Geometry: final body of the model. Coordinates: model frame, mm. Face numbers are marked on the shaded views. Give positions to 0.01 mm unless a question says otherwise; leave off trailing zeros. Order: outer loops, then holes, each group sorted by start corner. A loop starts at its lowest first (then second) coordinate and runs counter-clockwise, first axis right, second up. Notation, with made-up numbers: (39, -2.75) - (47, -2.75) arc R12 ccw to (47, 6.25) - close; hole circle Ø6 at (-28.75, 81.25). An arc over 180 degrees is marked (long way). Put each result on its own line as item: value. Start each with the question number.
1. Section A-A on x = 0. Return the cut outline in (y, z).
2. Section B-B on z = 0. Return the cut outline in (x, y).
3. Mould query, pull axis Z, two halves, no side actions, for the marked faces 1, 2 and 3. Classes: pulls with the +Z half, pulls with the -Z half, needs draft (parallel to the pull), parting line crosses it, or undercut.
4. Ray query, line 1 along X through (y, z) = (9.75, 0); line 2 along Y through (x, z) = (-4.5, 17); line 3 along Z through (x, y) = (30, 19). Return the intervals inside material, ascending. Write a range as from..to.
5. First-contact query: P1, Ø8, axis at y = 12, z = 2.5, coming from the +X side; P2, Ø2, axis at y = 17, z = -13, coming from the -X side; P3, Ø3, axis at x = -17, y = 2, coming from the +Z side. Flat tips, straight axial feed; report the tip coordinate or a pass-through.
6. Section C-C on y = 6.25. Return the cut outline in (x, z), plus the area to 3 significant figures.
from build123d import *

# Parameters (mm, degrees)
SKETCH1_R           = 35
SKETCH1_R_2         = 33
BOSS_EXTRUDE1_DEPTH = 25
EXTRUDE_START       = 3
SKETCH_1_R          = 35
EXTRUDE_1_DEPTH     = 3
CUT_EXTRUDE_START   = -10
SKETCH_3_R          = 35
SKETCH_3_R_2        = 34
CUT_EXTRUDE_1_DEPTH = 10
FILLET_1_R          = 1
FILLET_2_R          = 0.5


with BuildPart() as part:
    # Sketch1 → Boss-Extrude1 (new body)
    with BuildSketch(Plane(origin=(0, 0, 0), x_dir=(1, 0, 0), z_dir=(0, 1, 0))):
        with Locations(Location((0, 0, 0), (0, 0, 270))):
            Circle(SKETCH1_R)
        with Locations(Location((0, 0, 0), (0, 0, 270))):
            Circle(SKETCH1_R_2, mode=Mode.SUBTRACT)
    extrude(amount=BOSS_EXTRUDE1_DEPTH)

    # Эскиз1 → Бобышка-Вытянуть1 (add)
    with BuildSketch(Plane.XZ.offset(EXTRUDE_START)):
        with Locations(Location((0, 0, 0), (0, 0, 270))):
            Circle(SKETCH_1_R)
    extrude(amount=-EXTRUDE_1_DEPTH)

    # Эскиз3 → Вырез-Вытянуть1 (cut)
    with BuildSketch(Plane(origin=(0, 25, 0), x_dir=(1, 0, 0), z_dir=(0, 1, 0)).offset(CUT_EXTRUDE_START)):
        with Locations(Location((0, 0, 0), (0, 0, 90))):
            Circle(SKETCH_3_R)
        with Locations(Location((0, 0, 0), (0, 0, 270))):
            Circle(SKETCH_3_R_2, mode=Mode.SUBTRACT)
    extrude(amount=CUT_EXTRUDE_1_DEPTH, mode=Mode.SUBTRACT)

    # Скругление1
    fillet_1_edges = [part.edges().sort_by_distance(p)[0] for p in [
        (0, 0, -33),
    ]]
    fillet(fillet_1_edges, radius=FILLET_1_R)

    # Скругление2
    fillet_2_edges = [part.edges().sort_by_distance(p)[0] for p in [
        (0, -3, 35),
    ]]
    fillet(fillet_2_edges, radius=FILLET_2_R)


solid = part.part
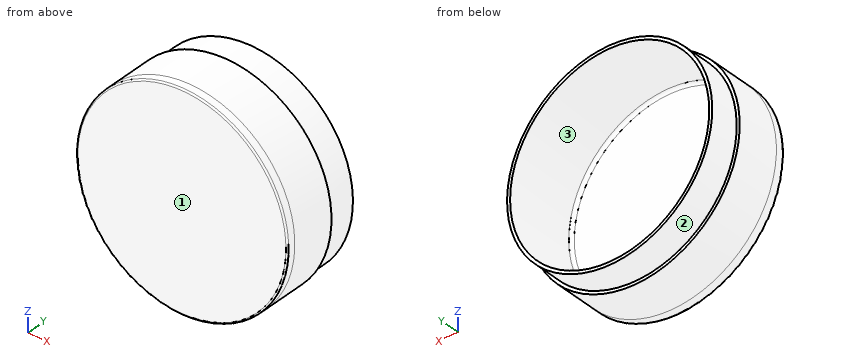
Resolved:
1. outline: (-3, -34.5) arc R0.5 ccw to (-2.5, -35) - (15, -35) - (15, -34) - (25, -34) - (25, -33) - (1, -33) arc R1 cw to (0, -32) - (0, 32) arc R1 cw to (1, 33) - (25, 33) - (25, 34) - (15, 34) - (15, 35) - (-2.5, 35) arc R0.5 ccw to (-3, 34.5) - close
2. outline: (-35, -2.5) arc R0.5 ccw to (-34.5, -3) - (34.5, -3) arc R0.5 ccw to (35, -2.5) - (35, 15) - (34, 15) - (34, 25) - (33, 25) - (33, 1) arc R1 cw to (32, 0) - (-32, 0) arc R1 cw to (-33, 1) - (-33, 25) - (-34, 25) - (-34, 15) - (-35, 15) - close
3. face 1: needs draft
3. face 2: parting line crosses it
3. face 3: undercut
4. line 1: -35..-33, 33..35
4. line 2: -3..0
4. line 3: -16..-13.75, 13.75..16
5. P1: x = 35
5. P2: x = -31.81
5. P3: z = 31.38
6. outline: circle Ø70 at (0, 0); hole circle Ø66 at (0, 0)
6. area: 427 mm^2
